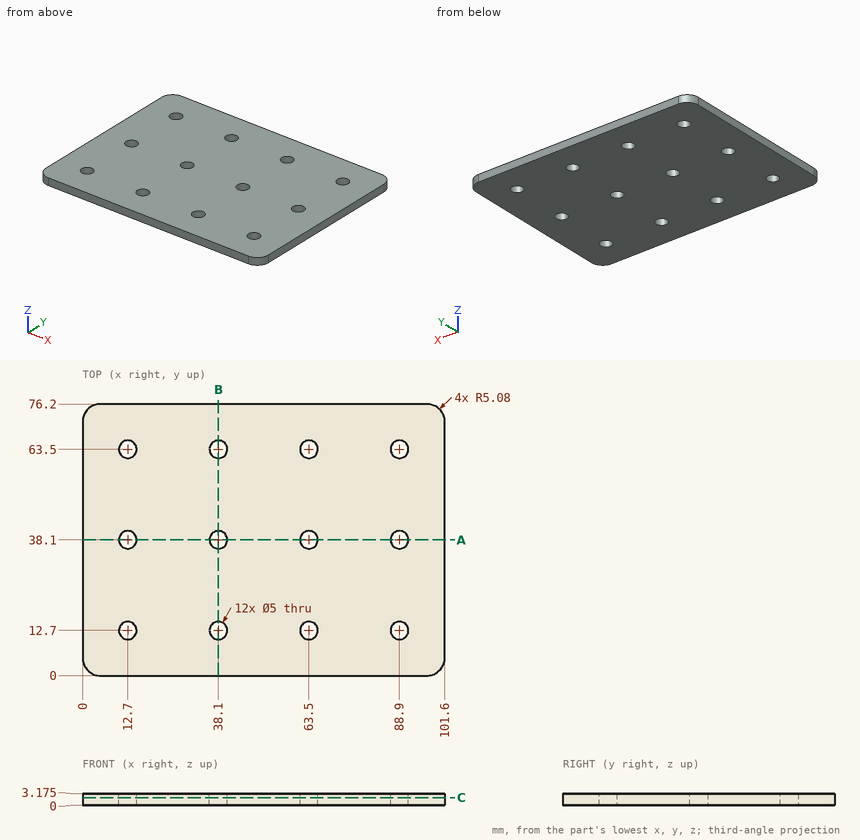
Answer from the drawing. Dimensions are ordinates in mm from the lowest x, y and z of the part. Give positions to 0.01 mm unless a question says otherwise; leave off trailing zeros. Loops run counter-clockwise (first coordinate to the right, second up) from the corner with the lowest first, then second, coordinate; pieces in that order, holes last. Notation, with made-up numbers: (48, 67.25) - (59, 67.25) arc R4 cw to (59, 72.25) - close; hole circle Ø9 at (28, 71). An arc over 180 degrees is marked (long way). Write each question's results on one line, items separated by ' | '.
1. Consider probe 1 along X at (y, z) = (13, 0.25); probe 2 along Y at (x, z) = (63.5, 2.5); probe 3 along Y at (x, z) = (63, 3). Determine where each line is inside the solid, lowest interval first. Write a range as from..to.
Resolved:
probe 1: x = 0..10.22, 15.18..35.62, 40.58..61.02, 65.98..86.42, 91.38..101.6 | probe 2: y = 0..10.2, 15.2..35.6, 40.6..61, 66..76.2 | probe 3: y = 0..10.25, 15.15..35.65, 40.55..61.05, 65.95..76.2
2. Find section B-B, the plane x = 38.1. Write down the section's boundary in (y, z) (3 decimals), then the cut area to 3 significant figures.
Resolved:
outline: (0, 0) - (10.2, 0) - (10.2, 3.175) - (0, 3.175) - close; (15.2, 0) - (35.6, 0) - (35.6, 3.175) - (15.2, 3.175) - close; (40.6, 0) - (61, 0) - (61, 3.175) - (40.6, 3.175) - close; (66, 0) - (76.2, 0) - (76.2, 3.175) - (66, 3.175) - close | area: 194 mm^2
3. Find section C-C, the plane z = 2.05. Count the separate pieces of the cut face and the enclosed holes in it, then the cut area to 3 significant figures.
Resolved:
separate pieces: 1 | enclosed holes: 12 | area: 7,480 mm^2
4. A flat-ended cylindrical pin translates along its axis: P1, Ø4, axis at x = 88.9, y = 38.1, coming from the -Z side (3 decimals). Find the tip coordinate at first contact, or state that the pin passes through.
Resolved:
P1: passes through
5. Find section A-A, the plane y = 38.1. Write down the section's boundary in (x, z) (3 decimals), then the cut area to 3 significant figures.
Resolved:
outline: (0, 0) - (10.2, 0) - (10.2, 3.175) - (0, 3.175) - close; (15.2, 0) - (35.6, 0) - (35.6, 3.175) - (15.2, 3.175) - close; (40.6, 0) - (61, 0) - (61, 3.175) - (40.6, 3.175) - close; (66, 0) - (86.4, 0) - (86.4, 3.175) - (66, 3.175) - close; (91.4, 0) - (101.6, 0) - (101.6, 3.175) - (91.4, 3.175) - close | area: 259 mm^2
